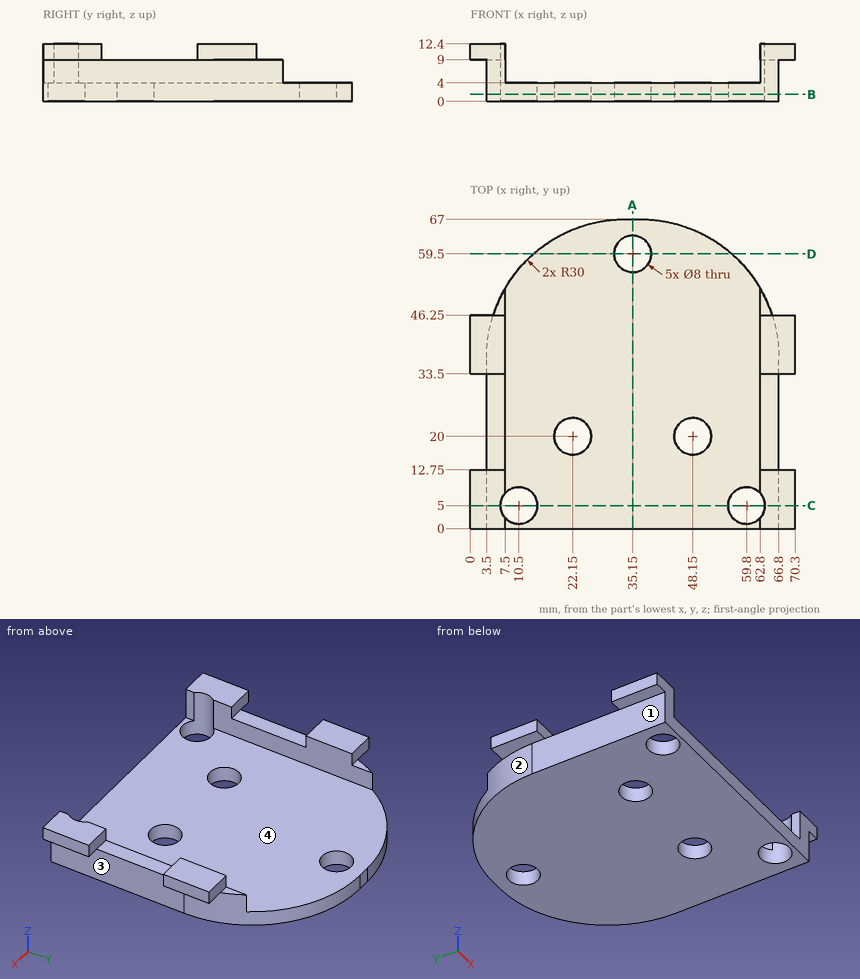
Can you work these out from the drawing? Everything is in mm from the part's minimum corner. A direction names the side the tool comes from. Give positions to 0.01 mm unless a question says otherwise; leave off trailing zeros. Order: outer loops, then holes, each group sorted by start corner. A loop starts at its lowest first (then second) coordinate and runs counter-clockwise, first axis right, second up. Notation, with made-up numbers: (1, 75.5) -> (36, 75.5) arc R10 cw to (36, 84.5) -> close; hole circle Ø2 at (-8.5, 84.5). An arc over 180 degrees is marked (long way). Return JSON: item names as keys, results as strings.
1. Imagine slicing it at A-A on x = 35.15. List the corners of the cut face in (y, z) for me.
Answer list:
{"outline": "(0, 0) -> (55.5, 0) -> (55.5, 4) -> (0, 4) -> close; (63.5, 0) -> (67, 0) -> (67, 4) -> (63.5, 4) -> close"}
2. For pin 1 Ø2 at (x, y) = (64, 28) entering from +Z; pin 2 Ø2.5 at (x, z) = (3.5, 10.5) entering from +Y; pin 3 Ø1.5 at (x, y) = (1.5, 37.5) entering from -Z, each with a flat end and sliding along its axis, tell me the tip position at first contact or that it passes through.
Answer list:
{"pin 1": "stops at z = 9", "pin 2": "stops at y = 46.25", "pin 3": "stops at z = 9"}
3. I need wall thicknesses on line 1 (X direction, y = 20, z = 1.6); line 2 (X direction, y = 5, z = 8.75); line 3 (Z direction, x = 61, y = 46). Which ranges of each line are inside material? Lowest first, please. Write a range as from..to.
Answer list:
{"line 1": "x = 3.5..18.15, 26.15..44.15, 52.15..66.8", "line 2": "x = 3.5..6.5, 63.8..66.8", "line 3": "z = 0..4"}
4. On a 3-axis mill with a long thin cutter (end or side, diameter ignored), from which of +Z, -Z, +X, -X, +Y, -Y can I reach the whole of each face in a straight line? I mean the marked faces 1, 2, 3 and 4. Say none if no direction works.
Answer list:
{"face 1": "-Z, -X, +Y, -Y", "face 2": "-Z, -X, +Y", "face 3": "-Z, +X, +Y, -Y", "face 4": "+Z, +Y, -Y"}
5. Imagine slicing it at D-D on y = 59.5. List the corners of the cut face in (x, z) for me.
Answer list:
{"outline": "(13.66, 0) -> (31.15, 0) -> (31.15, 4) -> (13.66, 4) -> close; (39.15, 0) -> (56.64, 0) -> (56.64, 4) -> (39.15, 4) -> close"}
6. Imagine slicing it at C-C on y = 5. List the corners of the cut face in (x, z) for me, then the cut area to 3 significant figures.
Answer list:
{"outline": "(0, 9) -> (3.5, 9) -> (3.5, 0) -> (6.5, 0) -> (6.5, 12.4) -> (0, 12.4) -> close; (14.5, 0) -> (55.8, 0) -> (55.8, 4) -> (14.5, 4) -> close; (63.8, 0) -> (66.8, 0) -> (66.8, 9) -> (70.3, 9) -> (70.3, 12.4) -> (63.8, 12.4) -> close", "area": "263 mm2"}
7. Imagine slicing it at B-B on z = 1.5. List the corners of the cut face in (x, y) for me, then the cut area to 3 significant figures.
Answer list:
{"outline": "(3.5, 0) -> (66.8, 0) -> (66.8, 37) arc R30 ccw to (36.8, 67) -> (33.5, 67) arc R30 ccw to (3.5, 37) -> close; hole circle Ø8 at (10.5, 5); hole circle Ø8 at (22.15, 20); hole circle Ø8 at (35.15, 59.5); hole circle Ø8 at (48.15, 20); hole circle Ø8 at (59.8, 5)", "area": "3,600 mm2"}
